```python
from build123d import *

# Parameters (mm, degrees)
SKETCH1_R           = 31.75
SKETCH1_R_2         = 4.7625
BOSS_EXTRUDE1_DEPTH = 27.94
SKETCH2_R           = 1.55575
BOSS_EXTRUDE2_DEPTH = 3.175
SKETCH3_R           = 19.05
CUT_EXTRUDE1_DEPTH  = 3.175


with BuildPart() as part:
    # Sketch1 → Boss-Extrude1 (new body)
    with BuildSketch(Plane(origin=(0, 0, 0), x_dir=(1, 0, 0), z_dir=(0, 1, 0))):
        with Locations(Location((0, 0, 0), (0, 0, 270))):
            Circle(SKETCH1_R)
        with Locations(Location((0, 0, 0), (0, 0, 270))):
            Circle(SKETCH1_R_2, mode=Mode.SUBTRACT)
    extrude(amount=BOSS_EXTRUDE1_DEPTH)

    # Sketch2 → Boss-Extrude2 (add)
    with BuildSketch(Plane(origin=(0, 27.94, 0), x_dir=(1, 0, 0), z_dir=(0, 1, 0))):
        with BuildLine():
            Line((-28.75, 31.75), (28.75, 31.75))
            ThreePointArc((28.75, 31.75), (30.871320344, 30.871320344), (31.75, 28.75))
            Line((31.75, 28.75), (31.75, -28.75))
            ThreePointArc((31.75, -28.75), (30.871320344, -30.871320344), (28.75, -31.75))
            Line((28.75, -31.75), (-28.75, -31.75))
            ThreePointArc((-28.75, -31.75), (-30.871320344, -30.871320344), (-31.75, -28.75))
            Line((-31.75, -28.75), (-31.75, 28.75))
            ThreePointArc((-31.75, 28.75), (-30.871320344, 30.871320344), (-28.75, 31.75))
        make_face()
        with Locations(Location((-26.940768363, 26.940768363, 0), (0, 0, 270))):
            Circle(SKETCH2_R, mode=Mode.SUBTRACT)
        with Locations(Location((26.940768363, 26.940768363, 0), (0, 0, 270))):
            Circle(SKETCH2_R, mode=Mode.SUBTRACT)
        with Locations(Location((26.940768363, -26.940768363, 0), (0, 0, 270))):
            Circle(SKETCH2_R, mode=Mode.SUBTRACT)
        with Locations(Location((-26.940768363, -26.940768363, 0), (0, 0, 270))):
            Circle(SKETCH2_R, mode=Mode.SUBTRACT)
    extrude(amount=BOSS_EXTRUDE2_DEPTH)

    # Sketch3 → Cut-Extrude1 (cut)
    with BuildSketch(Plane(origin=(0, 31.115, 0), x_dir=(1, 0, 0), z_dir=(0, 1, 0))):
        with Locations(Location((0, 0, 0), (0, 0, 270))):
            Circle(SKETCH3_R)
    extrude(amount=-CUT_EXTRUDE1_DEPTH, mode=Mode.SUBTRACT)


solid = part.part
```
The listing builds one solid part. Answer for the finished solid, in the listing's coordinates (mm). A direction names the side the tool comes from. Round coordinates to 2 decimals unless told otherwise and drop trailing zeros. Order: outer loops, then holes, each group sorted by start corner. A loop starts at its lowest first (then second) coordinate and runs counter-clockwise, first axis right, second up. Notation, with made-up numbers: (71, 78.5) -> (104, 78.5) arc R19 ccw to (104, 83.5) -> close; hole circle Ø6 at (-36, -37). An arc over 180 degrees is marked (long way). Answer as CSV lines item,"result".
Q1. A cutting plane is placed at C-C on z = -17. Determine the outline of the cut face in (x, y) (3 decimals).
Computed values:
outline,"(-31.75, 27.94) -> (-26.815, 27.94) -> (-26.815, 0) -> (26.815, 0) -> (26.815, 27.94) -> (31.75, 27.94) -> (31.75, 31.115) -> (8.597, 31.115) -> (8.597, 27.94) -> (-8.597, 27.94) -> (-8.597, 31.115) -> (-31.75, 31.115) -> close"
Q2. Which of the six approach directions +Z, -Z, +X, -X, +Y, -Y give full straight-line access (tool end or side, diameter ignored) to faces 4 (the cylindrical face through (-30.995, 13.774, -6.883)), 5 (the flat face through (24, 27.94, -25)), 6 (the cylindrical face through (26.345, 29.505, 28.378)), 7 (the flat face through (-4, 27.94, 4)), 8 (the flat face through (-7, 0, 0))?
Computed values:
face 4,"-Y"
face 5,"-Z, +X, -Y"
face 6,"+Y, -Y"
face 7,"+Y"
face 8,"+Z, -Z, +X, -X, -Y"
Q3. Consider line 1 (X direction, y = 30.2, z = 0); line 2 (Y direction, x = -12.5, z = 2); line 3 (Z direction, x = 14, y = 14.5). Determine where each line is inside the solid, lowest interval first. Write a range as from..to.
Computed values:
line 1,"x = -31.75..-19.05, 19.05..31.75"
line 2,"y = 0..27.94"
line 3,"z = -28.5..28.5"
Q4. Given pin 1 (5.5 mm diameter, centred on x = 0, z = 0, fed in from -Y); pin 2 (1 mm diameter, centred on y = 20, z = 11.5, fed in from +X); pin 3 (19 mm diameter, centred on x = -3.5, z = -3, fed in from +Y); pin 4 (5 mm diameter, centred on y = 3.5, z = 3.5, fed in from -X), each flat-ended and moving along its own axis, determine where each tip first touches the part or whether it passes through.
Computed values:
pin 1,"passes through"
pin 2,"stops at x = 29.78"
pin 3,"stops at y = 27.94"
pin 4,"stops at x = -31.73"
Q5. A cutting plane is placed at D-D on x = 11.5. Determine the outline of the cut face in (y, z) (3 decimals), plus the area to 3 significant figures.
Computed values:
outline,"(0, -29.594) -> (27.94, -29.594) -> (27.94, -31.75) -> (31.115, -31.75) -> (31.115, -15.187) -> (27.94, -15.187) -> (27.94, 15.187) -> (31.115, 15.187) -> (31.115, 31.75) -> (27.94, 31.75) -> (27.94, 29.594) -> (0, 29.594) -> close"
area,"1,760 mm^2"
Q6. For a pull along X with two mould halves and no side action, classify faces 1 (the cylindrical face through (30.85, 29.51, -30.89)), 2 (the cylindrical face through (-25.398, 29.505, -27.143)), 3 (the flat face through (-24, 27.94, -25)) as +X half, -X half, draft (parallel to the pull), parting line (faces both ways), or undercut.
Computed values:
face 1,"+X half"
face 2,"undercut"
face 3,"draft"
Q7. A cutting plane is placed at B-B on x = -4. Determine the outline of the cut face in (y, z) (3 decimals), plus the area to 3 significant figures.
Computed values:
outline,"(0, -31.497) -> (27.94, -31.497) -> (27.94, -31.75) -> (31.115, -31.75) -> (31.115, -18.625) -> (27.94, -18.625) -> (27.94, -2.585) -> (0, -2.585) -> close; (0, 2.585) -> (27.94, 2.585) -> (27.94, 18.625) -> (31.115, 18.625) -> (31.115, 31.75) -> (27.94, 31.75) -> (27.94, 31.497) -> (0, 31.497) -> close"
area,"1,700 mm^2"
